Here's how the part is built. I have some questions about the finished solid (model axes, mm). Round coordinates to 2 decimals unless told otherwise and drop trailing zeros. Order: outer loops, then holes, each group sorted by start corner. A loop starts at its lowest first (then second) coordinate and runs counter-clockwise, first axis right, second up. Notation, with made-up numbers: (5.25, 34.25) - (39.25, 34.25) arc R32 ccw to (39.25, 63.25) - close; hole circle Ø11 at (-32, -32.5). An arc over 180 degrees is marked (long way). One line per item, written item: value.
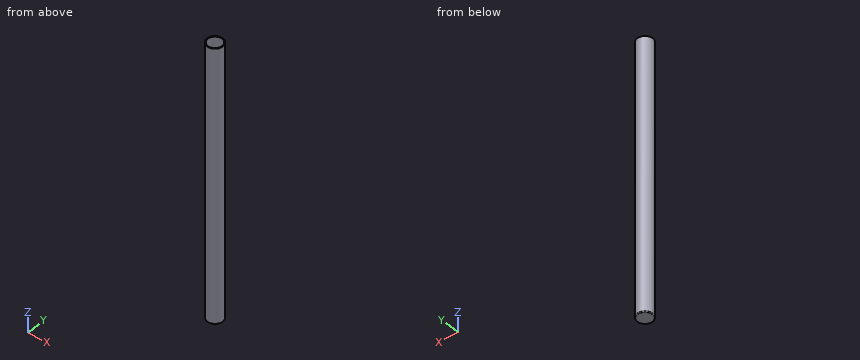
from build123d import *

# Parameters (mm, degrees)
F0_R     = 9
F1_DEPTH = 345
F2_T     = 1


# Not quite as in the source:
# - a fillet or chamfer that OpenCascade refuses, or shapes differently, is made with other operations: its cross-section is extruded or revolved along the edge and cut away or added


with BuildPart() as f1:
    # F0 (on Top) → F1 (new body)
    with BuildSketch(Plane.XY):
        Circle(F0_R)
    extrude(amount=-F1_DEPTH)

    # F2
    f2_openings = [f1.faces().sort_by_distance(p)[0] for p in [
        (0, 0, 0),
    ]]
    offset(amount=F2_T, openings=f2_openings, kind=Kind.INTERSECTION)

    # F3: fillet of radius 1 on 1 edges, made by hand

    # F3_s1 → F3_t2 (revolve, cut)
    with BuildSketch(Plane.XZ):
        with BuildLine():
            ThreePointArc((10, -345), (9.7071067812, -345.7071067812), (9, -346))
            Line((9, -346), (10, -346))
            Line((10, -346), (10, -345))
        make_face()
    revolve(axis=Axis((0, 0, -346), (0, 0, 1)), mode=Mode.SUBTRACT)


solid = f1.part
Q1. If we section it at A-A, the plane y = 0: Please give me the cut outline in (x, z).
Results list:
outline: (-10, -345) arc R1 ccw to (-9, -346) - (9, -346) arc R1 ccw to (10, -345) - (10, 0) - (9, 0) - (9, -345) - (-9, -345) - (-9, 0) - (-10, 0) - close
Q2. Will these pins go through, and if not, where does the flat tip stop? pin 1 (2 mm diameter, centred on x = -2, z = -235, fed in from -Y); pin 2 (2 mm diameter, centred on y = 3.5, z = -179, fed in from +X); pin 3 (6 mm diameter, centred on x = -7, z = -41.5, fed in from -Y).
Results list:
pin 1: y = -9.95
pin 2: x = 9.68
pin 3: y = -9.17
Q3. If I drill on line 1 along Y through (x, z) = (0.75, -292); line 2 along X through (y, z) = (-0.25, -243); line 3 along Y through (x, z) = (2, -300), over which ranges is the centre line in solid material (lowest first)?
Results list:
line 1: -9.97 to -8.97, 8.97 to 9.97
line 2: -10 to -9, 9 to 10
line 3: -9.8 to -8.77, 8.77 to 9.8
Q4. If we section it at C-C, the plane z = -281.5: Please give me the cut outline in (x, y).
Results list:
outline: circle Ø20 at (0, 0); hole circle Ø18 at (0, 0)
